Can you work these out from the model? Positions are in its coordinate system, mm. Face numbers are marked on the shaded views. Round coordinates to 2 decimals unless told otherwise and drop trailing zeros. Loops run counter-clockwise (first coordinate to the right, second up) from the corner with the lowest first, then second, coordinate; pieces in that order, holes last. Notation, with made-up numbers: (79, -8.75) -> (130, -8.75) arc R14 cw to (130, 18.25) -> close; hole circle Ø4 at (43.5, 85). An arc over 180 degrees is marked (long way). Write item = value, one per line.
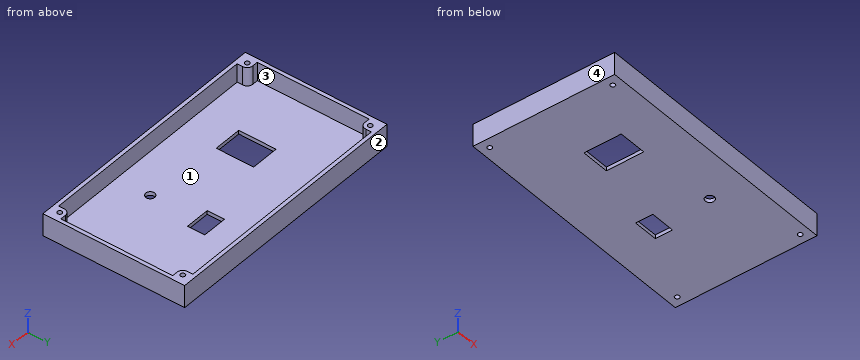
from build123d import *

# Parameters (mm, degrees)
SKETCH_W        = 136
SKETCH_H        = 76
PAD_DEPTH       = 2
SKETCH001_W     = 136
SKETCH001_H     = 76
PAD001_DEPTH    = 10
SKETCH002_R     = 1.25
POCKET_DEPTH    = 13
SKETCH003_R     = 2.375
SKETCH003_W     = 15.1
SKETCH003_H     = 20
SKETCH003_W_2   = 13.2
SKETCH003_H_2   = 9.2
POCKET001_DEPTH = 3
FILLET_R        = 3


with BuildPart() as part:
    # Sketch → Pad (new body)
    with BuildSketch(Plane.XY):
        Rectangle(SKETCH_W, SKETCH_H)
    extrude(amount=PAD_DEPTH)

    # Sketch001 (on Face6 of Pad) → Pad001 (join)
    with BuildSketch(Plane.XY.offset(2)):
        Rectangle(SKETCH001_W, SKETCH001_H)
        Polygon((-60, 36), (60, 36), (60, 30), (66, 30), (66, -30), (60, -30), (60, -36), (-60, -36), (-60, -30), (-66, -30), (-66, 30), (-60, 30), align=None, mode=Mode.SUBTRACT)
    extrude(amount=PAD001_DEPTH)

    # Sketch002 (on Face9 of Pad001) → Pocket (cut)
    with BuildSketch(Plane.XY.offset(12)):
        with Locations((-63, 33)):
            Circle(SKETCH002_R)
        with Locations((-63, -33)):
            Circle(SKETCH002_R)
        with Locations((63, 33)):
            Circle(SKETCH002_R)
        with Locations((63, -33)):
            Circle(SKETCH002_R)
    extrude(amount=-POCKET_DEPTH, mode=Mode.SUBTRACT)

    # Sketch003 (on Face4 of Pocket) → Pocket001 (cut)
    with BuildSketch(Plane(origin=(0, 0, 0), x_dir=(1, 0, 0), z_dir=(0, 0, -1))):
        with Locations((21, 18)):
            Circle(SKETCH003_R)
        with Locations((-28.06, 5.68)):
            Rectangle(SKETCH003_W, SKETCH003_H)
        with Locations((20.6, -11.6)):
            Rectangle(SKETCH003_W_2, SKETCH003_H_2)
    extrude(amount=-POCKET001_DEPTH, mode=Mode.SUBTRACT)

    # Fillet
    fillet_edges = [part.edges().sort_by_distance(p)[0] for p in [
        (60, 30, 7),
        (-60, 30, 7),
        (60, -30, 7),
        (-60, -30, 7),
    ]]
    fillet(fillet_edges, radius=FILLET_R)


solid = part.part
1. I'm going to push a flat-ended pin straight in: pin 1 (12 mm diameter, centred on x = -24.5, y = -1.5, fed in from -Z). Where does the tip first touch, or does it pass through?
Entries:
pin_1 = 0
2. Suppose I cut it at A-A, the plane y = -18. List the corners of the cut face in (x, z) for me (3 decimals), and give its area (4 significant figures).
Entries:
outline = (-68, 0) -> (18.625, 0) -> (18.625, 2) -> (-66, 2) -> (-66, 12) -> (-68, 12) -> close; (23.375, 0) -> (68, 0) -> (68, 12) -> (66, 12) -> (66, 2) -> (23.375, 2) -> close
area = 302.5 mm²
3. We'd pull the mould along X, two halves only. Please class the marked faces 1, 2, 3 and 4: released by +X, released by -X, zero draft, split by the parting line, or undercut.
Entries:
face_1 = undercut
face_2 = zero draft
face_3 = undercut
face_4 = released by -X
4. I need wall thicknesses on line 1 (Y direction, x = -63, z = 6); line 2 (X direction, y = -9, z = 9.75); line 3 (Y direction, x = 47, z = 5.5). Which ranges of each line are inside material? Lowest first, please. Write a range as [from, to].
Entries:
line_1 = [-38, -34.25], [-31.75, -30], [30, 31.75], [34.25, 38]
line_2 = [-68, -66], [66, 68]
line_3 = [-38, -36], [36, 38]
5. Suppose I cut it at C-C, the plane z = 10.5. List the corners of the cut face in (x, y) for me.
Entries:
outline = (-68, -38) -> (68, -38) -> (68, 38) -> (-68, 38) -> close; hole (-66, -30) -> (-63, -30) arc R3 cw to (-60, -33) -> (-60, -36) -> (60, -36) -> (60, -33) arc R3 cw to (63, -30) -> (66, -30) -> (66, 30) -> (63, 30) arc R3 cw to (60, 33) -> (60, 36) -> (-60, 36) -> (-60, 33) arc R3 cw to (-63, 30) -> (-66, 30) -> close; hole circle Ø2.5 at (-63, -33); hole circle Ø2.5 at (-63, 33); hole circle Ø2.5 at (63, -33); hole circle Ø2.5 at (63, 33)
6. Suppose I cut it at D-D, the plane y = 25.5. List the corners of the cut face in (x, z) for me, and give its area (3 significant figures).
Entries:
outline = (-68, 0) -> (68, 0) -> (68, 12) -> (66, 12) -> (66, 2) -> (-66, 2) -> (-66, 12) -> (-68, 12) -> close
area = 312 mm²
7. Suppose I cut it at B-B, the plane x = -24. List the corners of the cut face in (y, z) for me.
Entries:
outline = (-38, 0) -> (-15.68, 0) -> (-15.68, 2) -> (-36, 2) -> (-36, 12) -> (-38, 12) -> close; (4.32, 0) -> (38, 0) -> (38, 12) -> (36, 12) -> (36, 2) -> (4.32, 2) -> close
